For this review, take the finished solid that the model builds, in its own axes (mm). Face numbers are marked on the shaded views. A direction names the side the tool comes from. Coordinates: 2 decimals unless noted, no trailing zeros. Write each loop counter-clockwise with the first axis right and the second up, starting at its lowest first coordinate (ties: lowest second). Pieces come first, ordered by that corner, then holes. Notation, with made-up numbers: (-17.5, -2.5) -> (9.5, -2.5) arc R27 cw to (9.5, 15.5) -> close; hole circle Ø10 at (79, 5.25). An arc over 180 degrees is marked (long way). Put each result on its own line as item: value. Start each with the question number.
Item 1: Consider section A-A on y = 3. Give the boundary of the cut face in (x, z), and give its area (3 significant figures).
Item 2: Consider section C-C on z = -8. Give the boundary of the cut face in (x, y).
Item 3: The part is to be moulded in two halves that separate along Z. For the marked faces 1, 2, 3 and 4, say which applies: +Z half, -Z half, draft (parallel to the pull), parting line (faces both ways), or undercut.
Item 4: Consider section B-B on x = -3. Give the boundary of the cut face in (y, z), and give its area (3 significant figures).
Item 5: Insertion check: P1, Ø4, axis at x = 0, z = 0, coming from the +Y side; P2, Ø2.5, axis at x = -20, z = 0, coming from the +Y side; P3, Ø3, axis at x = -4.5, z = 13.5, coming from the +Y side. Each pin has a flat end and moves straight along its axis. Give the tip position at first contact, or say it passes through.
Item 6: To check wall thickness, follow L1, parallel to X at y = -1.35, z = 0; L2, parallel to Z at x = -20, y = -0.9; L3, parallel to Y at x = 9.5, z = -4.5. State the ranges of each line that lie inside material, in increasing order.
Item 7: For the marked faces 5 and 6, list the 3-axis set-ups (+Z, -Z, +X, -X, +Y, -Y) from which the entire face can be reached by the end or side of a thin tool; tool diameter is ignored.
```python
from build123d import *

# Parameters (mm, degrees)
SKETCH1_W           = 60
SKETCH1_H           = 40
BOSS_EXTRUDE1_DEPTH = 10
SKETCH1_3_W         = 60
SKETCH1_3_H         = 40
SKETCH1_3_R         = 1.5
BOSS_EXTRUDE2_DEPTH = 2


with BuildPart() as part:
    # Sketch1 → Boss-Extrude1 (new body)
    with BuildSketch(Plane(origin=(0, 0, 0), x_dir=(1, 0, 0), z_dir=(0, 1, 0))):
        with Locations((-10, 0)):
            Rectangle(SKETCH1_W, SKETCH1_H)
        with BuildLine():
            ThreePointArc((-20, 14), (-34, 0), (-20, -14))
            Line((-20, -14), (0, -14))
            ThreePointArc((0, -14), (14, 0), (0, 14))
            Line((0, 14), (-20, 14))
        make_face(mode=Mode.SUBTRACT)
    extrude(amount=BOSS_EXTRUDE1_DEPTH)

    # Sketch1_3 → Boss-Extrude2 (add)
    with BuildSketch(Plane(origin=(0, 0, 0), x_dir=(1, 0, 0), z_dir=(0, 1, 0))):
        with Locations((-10, 0)):
            Rectangle(SKETCH1_3_W, SKETCH1_3_H)
        with BuildLine():
            ThreePointArc((-20, 14), (-34, 0), (-20, -14))
            Line((-20, -14), (0, -14))
            ThreePointArc((0, -14), (14, 0), (0, 14))
            Line((0, 14), (-20, 14))
        make_face(mode=Mode.SUBTRACT)
        with BuildLine():
            Line((-20, 14), (0, 14))
            ThreePointArc((0, 14), (14, 0), (0, -14))
            Line((0, -14), (-20, -14))
            ThreePointArc((-20, -14), (-34, 0), (-20, 14))
        make_face()
        with Locations((-20, 0)):
            Circle(SKETCH1_3_R, mode=Mode.SUBTRACT)
        Circle(SKETCH1_3_R, mode=Mode.SUBTRACT)
    extrude(amount=-BOSS_EXTRUDE2_DEPTH)


solid = part.part
```
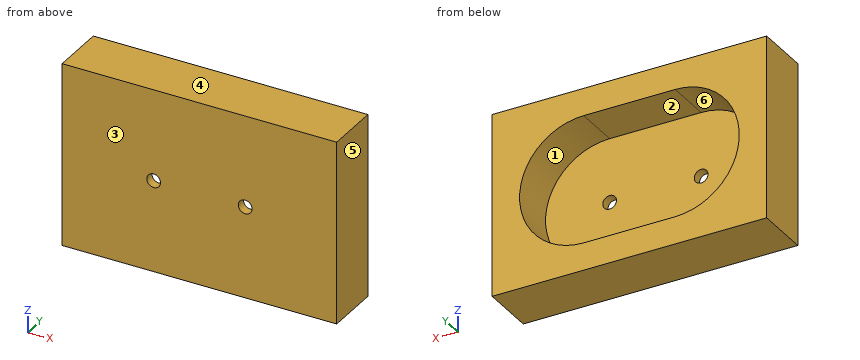
Return value:
1. outline: (-40, -20) -> (20, -20) -> (20, 20) -> (-40, 20) -> close; hole (-20, -14) -> (0, -14) arc R14 ccw to (0, 14) -> (-20, 14) arc R14 ccw to start
1. area: 1,220 mm^2
2. outline: (-40, -2) -> (20, -2) -> (20, 10) -> (11.49, 10) -> (11.49, 0) -> (-31.49, 0) -> (-31.49, 10) -> (-40, 10) -> close
3. face 1: undercut
3. face 2: undercut
3. face 3: draft
3. face 4: +Z half
4. outline: (-2, -20) -> (10, -20) -> (10, -14) -> (0, -14) -> (0, 14) -> (10, 14) -> (10, 20) -> (-2, 20) -> close
4. area: 200 mm^2
5. P1: y = 0
5. P2: through
5. P3: y = 10
6. L1: -40 to -21.5, -18.5 to -1.5, 1.5 to 20
6. L2: -20 to -1.5, 1.5 to 20
6. L3: -2 to 0
7. face 5: +Z, -Z, +X, +Y, -Y
7. face 6: +Y
